Autodesk Inventor part; units mm, degrees
ref_plane "YZ Plane" through (0, 0, 0) normal (1, 0, 0) x (0, 1, 0)
ref_plane "XZ Plane" through (0, 0, 0) normal (0, 1, 0) x (-1, 0, 0)
ref_plane "XY Plane" through (0, 0, 0) normal (0, 0, 1) x (1, 0, 0)
sketch "スケッチ2" plane through (0, 0, 0) normal (1, 0, 0) x (0, 1, 0)
  line L0 (-50, 46.625) -> (0, 46.625)
  line L1 (0, 46.625) -> (0, 36.625)
  line L2 (0, 36.625) -> (-50, 36.625)
  line L3 (-50, 36.625) -> (-50, 46.625)
  line L4 (0, 36.625) -> (-8, 36.625)
  line L5 (-8, 36.625) -> (-8, 0)
  line L6 (-8, 0) -> (0, 0)
  line L7 (0, 0) -> (0, 36.625)
  circle A0 centre (-20, 41.625) radius 2.25
  circle A1 centre (-35, 41.625) radius 2.25
  line L8 (-8, 36.625) -> (0, 36.625)
  line L9 (0, 36.625) -> (0, 54)
  line L10 (0, 54) -> (-8, 54)
  line L11 (-8, 54) -> (-8, 36.625)
  point P0 (-8, 46.625)
  point P1 (0, 46.625)
  dimension "d7" = 50
  dimension "d8" = 10
  dimension "d10" = 8
  dimension "d11" = 4.5
  dimension "d12" = 4.5
  dimension "d13" = 15
  dimension "d14" = 20
  dimension "d15" = 5
  dimension "d16" = 5
  dimension "d27" = 54
  dimension "d28" = 7.375
extrude "押し出し2" add sketch "スケッチ2" along normal blind 6 contours L0 L11 L2 L3
extrude "押し出し5" add sketch "スケッチ2" along normal blind 70 contours L11 L10 L9 L0 | L0 L1 L2 L11 | L2 L7 L6 L5
sketch "スケッチ4" plane through (0, -8, 0) normal (0, -1, 0) x (1, 0, 0)
  line L0 (70, 0) -> (70, 54)
  line L1 (70, 15) -> (15, 0)
  line L2 (15, 0) -> (15, 54)
  line L3 (15, 54) -> (70, 39)
  line L4 (0, 54) -> (70, 54)
  line L5 (0, 36.625) -> (0, 0)
  line L6 (0, 0) -> (70, 0)
  line L7 (0, 25.077) -> (7.9173, 25.077)
  line L8 (7.9173, 25.077) -> (7.9173, 0)
  line L9 (7.9173, 0) -> (0, 0)
  line L10 (0, 0) -> (0, 25.077)
  dimension "d31" = 15
  dimension "d32" = 15
  dimension "d33" = 15
extrude "押し出し6" cut sketch "スケッチ4" against normal blind 8 contours L6 L1 L0 | L6 L5 L7 L8 | L3 L4 L0
sketch "スケッチ5" plane through (0, 0, 54) normal (0, 1, 0) x (1, 0, 0)
  line L0 (15, 0) -> (70, 15)
  line L1 (70, 39) -> (15, 54)
  line L2 (70.01, 38.9973) -> (70.01, 15.0027)
  line L3 (70, 15) -> (15, 0)
  line L4 (70, 39) -> (70, 15)
  line L5 (70.01, 15.0027) -> (70, 15)
  line L6 (70.01, 38.9973) -> (70, 39)
  point P0 (0, 54)
  dimension "d37" = 0.01
extrude "押し出し7" add sketch "スケッチ5" against normal blind 8
properties part number "left-nail" material "ABS プラスチック"
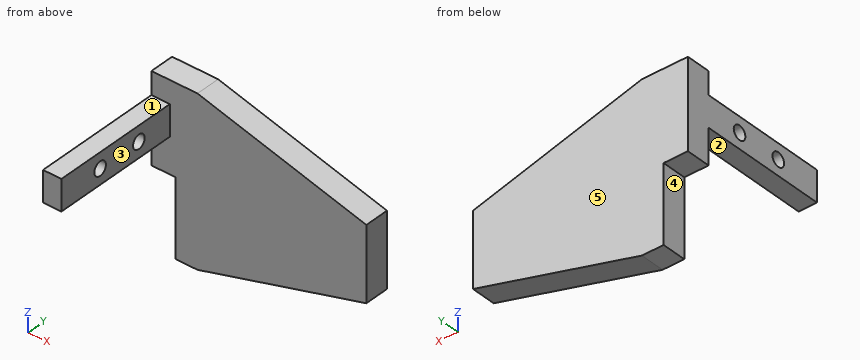
The listing builds one solid part. Answer for the finished solid, in the listing's coordinates (mm). Face numbers are marked on the shaded views. A direction names the side the tool comes from. Give positions to 0.01 mm unless a question says otherwise; leave off trailing zeros. Write each loop counter-clockwise with the first axis right and the second up, starting at its lowest first coordinate (ties: lowest second). Pieces come first, ordered by that corner, then holes.
Item 1: Section B-B, the plane z = 45 is taken. Write down the section's boundary in (x, y), plus the area to 3 significant figures.
Item 2: Find the intervals of material crossed by line 1 along Z through (x, y) = (4.75, -35) (3 decimals); line 2 along Y through (x, z) = (27, 42); line 3 along X through (y, z) = (-21.5, 38.5), in increasing order.
Item 3: Section D-D, the plane z = 33.5 is taken. Write down the section's boundary in (x, y).
Item 4: Section A-A, the plane y = -20 is taken. Write down the section's boundary in (x, z) (3 decimals).
Item 5: Flat-ended cylindrical pins translate along their axes: P1, Ø5, axis at x = 2, y = -39, coming from the +Z side (3 decimals); P2, Ø3, axis at x = 2, y = -33.5, coming from the -Z side (3 decimals); P3, Ø8, axis at y = -24, z = 32.5, coming from the -X side; P4, Ø3, axis at x = 54, y = -6.5, coming from the +Z side. Find the tip coordinate at first contact, or state that the pin passes through.
Item 6: Which of the six approach directions +Z, -Z, +X, -X, +Y, -Y give full straight-line access (tool end or side, diameter ignored) to the marked faces 1, 2, 3, 4 and 5?
Item 7: Section C-C, the plane y = -27.5 is taken. Write down the section's boundary in (x, z) (3 decimals).
Completed:
1. outline: (0, -50) - (6, -50) - (6, -8) - (48, -8) - (48, 0) - (0, 0) - close
1. area: 636 mm2
2. line 1: z = 36.625 to 39.375, 43.875 to 46.625
2. line 2: y = -8 to 0
2. line 3: x = 0 to 6
3. outline: (0, -8) - (70.01, -8) - (70.01, 0) - (0, 0) - close
4. outline: (0, 36.625) - (6, 36.625) - (6, 39.375) - (0, 39.375) - close; (0, 43.875) - (6, 43.875) - (6, 46.625) - (0, 46.625) - close
5. P1: stops at z = 46.625
5. P2: stops at z = 36.625
5. P3: passes through
5. P4: stops at z = 43.77
6. face 1: +Z, +X, -X, -Y
6. face 2: -Z, +X, -X, -Y
6. face 3: +Z, -Z, +X, -Y
6. face 4: -Z, -X, +Y, -Y
6. face 5: +Z, -Z, +X, -X, +Y
7. outline: (0, 36.625) - (6, 36.625) - (6, 46.625) - (0, 46.625) - close
